Here's how the part is built. I have some questions about the finished solid (model axes, mm). Face numbers are marked on the shaded views. A direction names the side the tool comes from. Round coordinates to 2 decimals unless told otherwise and drop trailing zeros. Write each loop counter-clockwise with the first axis right and the second up, starting at its lowest first coordinate (ties: lowest second). Pieces come first, ordered by that corner, then holes. Notation, with made-up numbers: (85, 49) - (127, 49) arc R16 cw to (127, 69) - close; hole circle Ø7 at (33.25, 48). An arc over 180 degrees is marked (long way). One line per item, written item: value. Start each with the question number.
Item 1: Imagine slicing it at B-B, the plane y = 5. Please give me the cut outline in (x, z), then the cut area to 3 significant figures.
Item 2: Imagine slicing it at A-A, the plane x = 52.5. Please give me the cut outline in (y, z), then the cut area to 3 significant figures.
Item 3: Imagine slicing it at D-D, the plane x = 82. Please give me the cut outline in (y, z).
Item 4: For the marked faces 1, 2, 3, 4 and 5, which set-ups out of +Z, -Z, +X, -X, +Y, -Y let a thin tool reach every point of the face, with its end or its side?
Item 5: For P1, Ø1, axis at x = 71.5, y = -21.5, coming from the +Z side; P2, Ø10, axis at y = 17, z = 6, coming from the +X side; P3, Ø9.5, axis at y = -0.5, z = 12.5, coming from the -X side, each with a flat end and sliding along its axis, tell me the tip position at first contact or that it passes through.
Item 6: If I drill on line 1 (Y direction, x = 41.5, z = 8); line 2 (Y direction, x = 62, z = 18.5); line 3 (Y direction, x = 17, z = 5.15), over which ranges is the centre line in solid material (lowest first)?
Item 7: Thinking about a two-plate mould opening in Y: for the marked faces 6, 7 and 8, which applies, released by +Y, released by -Y, zero draft, split by the parting line, or undercut?
```python
from build123d import *

# Parameters (mm, degrees)
SKETCH_R          = 1.6
PAD_DEPTH         = 21
POCKET_DEPTH      = 36.1638711749
POCKET_DEPTH_BACK = 36.1638711749
POCKET001_DEPTH   = 3
POCKET002_DEPTH   = 12
SKETCH004_R       = 3
POCKET003_DEPTH   = 3
SKETCH005_R       = 3
POCKET004_DEPTH   = 3
POCKET005_DEPTH   = 30.8
POCKET006_DEPTH   = 4
POCKET007_DEPTH   = 18


with BuildPart() as part:
    # Sketch → Pad (new body)
    with BuildSketch(Plane.XY):
        with BuildLine():
            ThreePointArc((0.9, 21.6), (0.2250976252, 10.8093709323), (0, 0))
            ThreePointArc((0, 0), (0.2250976252, -10.8093709323), (0.9, -21.6))
            ThreePointArc((0.9, -21.6), (4.7770016669, -30.6223150598), (13.3, -35.5))
            ThreePointArc((13.3, -35.5), (16.6336444708, -35.9967498287), (20, -36.1628711749))
            Line((20, -36.1628711749), (64.2, -36.1628711749))
            ThreePointArc((64.2, -36.1628711749), (80.950441462, -30.2745268069), (90.3317276275, -15.2))
            ThreePointArc((90.3317276275, -15.2), (91.5816834036, -7.6456381799), (92, 0))
            ThreePointArc((92, 0), (91.5816834036, 7.6456381799), (90.3317276275, 15.2))
            ThreePointArc((90.3317276275, 15.2), (80.950441462, 30.2745268069), (64.2, 36.1628711749))
            Line((20, 36.1628711749), (64.2, 36.1628711749))
            ThreePointArc((20, 36.1628711749), (16.6336444708, 35.9967498287), (13.3, 35.5))
            ThreePointArc((13.3, 35.5), (4.7770016669, 30.6223150598), (0.9, 21.6))
        make_face()
        with Locations((17, 25)):
            Circle(SKETCH_R, mode=Mode.SUBTRACT)
        with Locations((17, -25)):
            Circle(SKETCH_R, mode=Mode.SUBTRACT)
        with BuildLine():
            ThreePointArc((83.6, 0), (82, 1.6), (80.4, 0))
            ThreePointArc((80.4, 0), (82, -1.6), (83.6, 0))
        make_face(mode=Mode.SUBTRACT)
        Polygon((23.3, 0), (23.3, 22.4), (59.9, 22.4), (59.9, 10.5), (72.1, 10.5), (72.1, 0), (72.1, -10.5), (59.9, -10.5), (59.9, -22.4), (23.3, -22.4), align=None, mode=Mode.SUBTRACT)
    extrude(amount=PAD_DEPTH)

    # Sketch001 → Pocket (cut, two sides)
    with BuildSketch(Plane.XZ) as pocket_sk:
        with BuildLine():
            Line((0, 5), (0, 21))
            Line((0, 21), (20, 21))
            ThreePointArc((20, 21), (18.9362470202, 20.6928206855), (18.2, 19.8658564429))
            Line((18.2, 19.8658564429), (11.9, 6.7))
            ThreePointArc((10.6, 5.6), (11.3678698195, 6.0106993043), (11.9, 6.7))
            ThreePointArc((8, 5.008391541), (9.3083281759, 5.267595115), (10.6, 5.6))
            ThreePointArc((7.9, 5), (7.9501757361, 5.0021015655), (8, 5.008391541))
            Line((0, 5), (7.9, 5))
        make_face()
    extrude(amount=-POCKET_DEPTH, mode=Mode.SUBTRACT)
    extrude(pocket_sk.sketch, amount=POCKET_DEPTH_BACK, mode=Mode.SUBTRACT)

    # Sketch002 (on Face34 of Pocket) → Pocket001 (cut)
    with BuildSketch(Plane.XY.offset(21)):
        with BuildLine():
            Line((24.2, 30.78), (0, 30.78))
            Line((0, 0), (0, 30.78))
            Line((0, 0), (0, -30.78))
            Line((24.2, -30.78), (0, -30.78))
            Line((24.2, -30.78), (24.2, -28.88))
            ThreePointArc((25.4, -27.68), (24.5514718626, -28.0314718626), (24.2, -28.88))
            Line((25.4, -27.68), (70.2, -27.68))
            ThreePointArc((70.2, -27.68), (77.4415537007, -26.3958494637), (83.8, -22.7))
            ThreePointArc((83.8, -22.7), (86.8411272784, -19.0996370304), (88.5305835924, -14.7))
            ThreePointArc((88.5305835924, -14.7), (89.6317327981, -7.3866295524), (90, 0))
            ThreePointArc((90, 0), (89.6317327981, 7.3866295524), (88.5305835924, 14.7))
            ThreePointArc((88.5305835924, 14.7), (86.8411272784, 19.0996370304), (83.8, 22.7))
            ThreePointArc((83.8, 22.7), (77.4415537007, 26.3958494637), (70.2, 27.68))
            Line((25.4, 27.68), (70.2, 27.68))
            ThreePointArc((24.2, 28.88), (24.5514718626, 28.0314718626), (25.4, 27.68))
            Line((24.2, 30.78), (24.2, 28.88))
        make_face()
    extrude(amount=-POCKET001_DEPTH, mode=Mode.SUBTRACT)

    # Sketch003 (on Face35 of Pocket001) → Pocket002 (cut)
    with BuildSketch(Plane.XY.offset(18)):
        with BuildLine():
            Line((0, 0), (0, 30.78))
            Line((0, 30.78), (24.2, 30.78))
            Line((24.2, 28.88), (24.2, 30.78))
            ThreePointArc((24.2, 28.88), (24.5514718626, 28.0314718626), (25.4, 27.68))
            Line((25.4, 27.68), (70.2, 27.68))
            ThreePointArc((73.4, 27.4354687069), (71.8046647277, 27.6187781914), (70.2, 27.68))
            Line((73.4, 27.4354687069), (73.4, 0))
            Line((73.4, -27.4354687069), (73.4, 0))
            ThreePointArc((70.2, -27.68), (71.8046647277, -27.6187781914), (73.4, -27.4354687069))
            Line((25.4, -27.68), (70.2, -27.68))
            ThreePointArc((25.4, -27.68), (24.5514718626, -28.0314718626), (24.2, -28.88))
            Line((24.2, -28.88), (24.2, -30.78))
            Line((0, -30.78), (24.2, -30.78))
            Line((0, 0), (0, -30.78))
        make_face()
    extrude(amount=-POCKET002_DEPTH, mode=Mode.SUBTRACT)

    # Sketch004 (on Face39 of Pocket002) → Pocket003 (cut)
    with BuildSketch(Plane.XY.offset(6)):
        with Locations((17, 25)):
            Circle(SKETCH004_R)
        with Locations((17, -25)):
            Circle(SKETCH004_R)
    extrude(amount=-POCKET003_DEPTH, mode=Mode.SUBTRACT)

    # Sketch005 (on Face42 of Pocket003) → Pocket004 (cut)
    with BuildSketch(Plane.XY.offset(18)):
        with Locations((82, 0)):
            Circle(SKETCH005_R)
    extrude(amount=-POCKET004_DEPTH, mode=Mode.SUBTRACT)

    # Sketch006 → Pocket005 (cut, symmetric)
    with BuildSketch(Plane.XZ):
        Polygon((73.4, 15), (51, 15), (48.5, 16), (25, 16), (24.2, 16.4), (24.2, 6), (73.4, 6), align=None)
    extrude(amount=POCKET005_DEPTH, both=True, mode=Mode.SUBTRACT)

    # Sketch007 (on Face2 of Pocket005) → Pocket006 (cut)
    with BuildSketch(Plane(origin=(0, 0, 0), x_dir=(1, 0, 0), z_dir=(0, 0, -1))):
        Polygon((21.3, 0), (21.3, 12.5), (23.3, 12.5), (23.3, 24.5), (62.3, 24.5), (62.3, 12.5), (75.3, 12.5), (75.3, 0), (75.3, -12.5), (62.3, -12.5), (62.3, -24.5), (23.3, -24.5), (23.3, -12.5), (21.3, -12.5), align=None)
    extrude(amount=-POCKET006_DEPTH, mode=Mode.SUBTRACT)

    # Sketch008 → Pocket007 (cut, symmetric)
    with BuildSketch(Plane.XZ):
        Polygon((5.5, 0), (11, 0), (11, 2), (16.7, 6), (4.45, 6), (4.45, 5), (5.5, 3.5), align=None)
    extrude(amount=POCKET007_DEPTH, both=True, mode=Mode.SUBTRACT)


solid = part.part
```
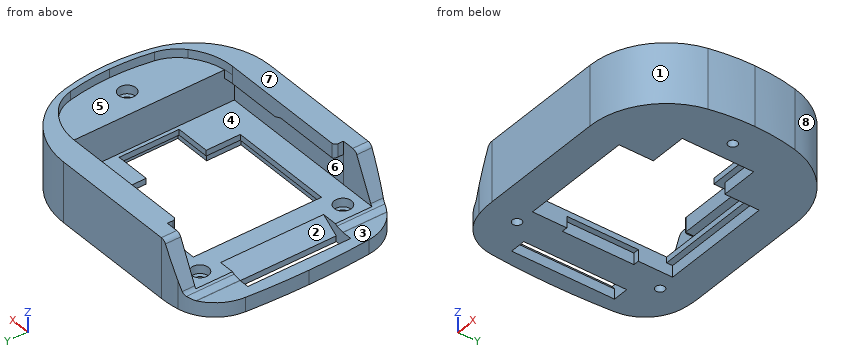
Values follow:
1. outline: (0.05, 0) - (5.5, 0) - (5.5, 3.5) - (4.45, 5) - (0.05, 5) - close; (11, 0) - (21.3, 0) - (21.3, 4) - (23.3, 4) - (23.3, 6) - (16.7, 6) - (11, 2) - close; (72.1, 4) - (75.3, 4) - (75.3, 0) - (91.82, 0) - (91.82, 21) - (89.83, 21) - (89.83, 18) - (73.4, 18) - (73.4, 6) - (72.1, 6) - close
1. area: 413 mm^2
2. outline: (-36.16, 0) - (-24.5, 0) - (-24.5, 4) - (-22.4, 4) - (-22.4, 6) - (-30.8, 6) - (-30.8, 15) - (-27.68, 15) - (-27.68, 21) - (-36.16, 21) - close; (22.4, 4) - (24.5, 4) - (24.5, 0) - (36.16, 0) - (36.16, 21) - (27.68, 21) - (27.68, 15) - (30.8, 15) - (30.8, 6) - (22.4, 6) - close
2. area: 347 mm^2
3. outline: (-29.39, 0) - (-1.6, 0) - (-1.6, 15) - (-3, 15) - (-3, 18) - (-24.06, 18) - (-24.06, 21) - (-29.39, 21) - close; (1.6, 0) - (29.39, 0) - (29.39, 21) - (24.06, 21) - (24.06, 18) - (3, 18) - (3, 15) - (1.6, 15) - close
4. face 1: +Z, -Z, +X, -Y
4. face 2: +Z
4. face 3: +Z, -X, +Y, -Y
4. face 4: -X
4. face 5: +Z, -X
5. P1: stops at z = 6
5. P2: stops at x = 90.96
5. P3: stops at x = 73.4
6. line 1: y = -36.16 to -30.8, 30.8 to 36.16
6. line 2: y = -36.16 to -27.68, 27.68 to 36.16
6. line 3: y = -36.03 to -28, -22 to 22, 28 to 36.03
7. face 6: undercut
7. face 7: zero draft
7. face 8: released by +Y
